Geometry: final body of the model. Coordinates: model frame, mm. A direction names the side the tool comes from. Round coordinates to 2 decimals unless told otherwise and drop trailing zeros. Loops run counter-clockwise (first coordinate to the right, second up) from the corner with the lowest first, then second, coordinate; pieces in that order, holes last. Notation, with made-up numbers: (-38, -13.5) - (-19, -13.5) arc R28 cw to (-19, 20.5) - close; hole circle Ø2 at (-27, -39.75). An arc over 180 degrees is marked (long way). Answer as a JSON object with one key per item and string values. Group by question number.
Item 1: Section B-B (z = 32). Return the cut outline in (x, y).
Item 2: Draft query along Y for faces 1 (the face through (-22.804, 25.315, 2.994)), 2 (the face through (-22.804, 21.115, 2.994)), 3 (the face through (-39.05, 1.97, -8.67)), 4 (the face through (0, 4, 3)). Return one class per face: released by +Y, released by -Y, zero draft, split by the parting line, or undercut.
Item 3: Section A-A (y = 7.25). Return the cut outline in (x, z).
Item 4: Line query: line 1 (X direction, y = 8.5, z = 0); line 2 (X direction, y = 1, z = 0); line 3 (Y direction, x = -6, z = -22.5). Output: solid intervals per line, ascending.
Item 5: First-contact query: pin 1 (3 mm diameter, centred on y = 14, z = 16.5, fed in from -X); pin 2 (3 mm diameter, centred on y = 19.5, z = -3.5, fed in from +X); pin 3 (16 mm diameter, centred on x = 0, z = 0, fed in from +Y). Flat tips, straight axial feed; report the tip coordinate or a pass-through.
Item 6: Reachability of faces 5 (the face through (7.21, 27.19, 22.89)), 6 (the face through (-12.93, 30, 11.3)) from +Z, -Z, +X, -X, +Y, -Y: full face, straight path, thin tool, end or side. Return the list, or none.
```python
from build123d import *

# Parameters (mm, degrees)
SKETCH1_R           = 40
SKETCH1_R_2         = 2.1
BOSS_EXTRUDE1_DEPTH = 4
SKETCH2_R           = 25
SKETCH2_R_2         = 6.1
BOSS_EXTRUDE5_DEPTH = 9
SKETCH6_R           = 22
SKETCH6_R_2         = 17
BOSS_EXTRUDE6_DEPTH = 5
SKETCH7_R           = 24
SKETCH7_R_2         = 17
BOSS_EXTRUDE7_DEPTH = 12
SKETCH9_W           = 1
SKETCH9_H           = 2.2
CHAMFER1_SIZE       = 2
FILLET1_R           = 2


with BuildPart() as part:
    # Sketch1 → Boss-Extrude1 (new body)
    with BuildSketch(Plane(origin=(0, 0, 0), x_dir=(1, 0, 0), z_dir=(0, 1, 0))):
        with Locations(Location((0, 0, 0), (0, 0, 270))):
            Circle(SKETCH1_R)
        with Locations(Location((0, 0, 0), (0, 0, 270))):
            Circle(SKETCH1_R_2, mode=Mode.SUBTRACT)
    extrude(amount=BOSS_EXTRUDE1_DEPTH)

    # Sketch2 → Boss-Extrude5 (add)
    with BuildSketch(Plane(origin=(0, 4, 0), x_dir=(1, 0, 0), z_dir=(0, 1, 0))):
        with Locations(Location((0, 0, 0), (0, 0, 270))):
            Circle(SKETCH2_R)
        with Locations(Location((0, 0, 0), (0, 0, 270))):
            Circle(SKETCH2_R_2, mode=Mode.SUBTRACT)
    extrude(amount=BOSS_EXTRUDE5_DEPTH)

    # Sketch6 → Boss-Extrude6 (add)
    with BuildSketch(Plane(origin=(0, 13, 0), x_dir=(1, 0, 0), z_dir=(0, 1, 0))):
        with Locations(Location((0, 0, 0), (0, 0, 270))):
            Circle(SKETCH6_R)
        with Locations(Location((0, 0, 0), (0, 0, 270))):
            Circle(SKETCH6_R_2, mode=Mode.SUBTRACT)
    extrude(amount=BOSS_EXTRUDE6_DEPTH)

    # Sketch7 → Boss-Extrude7 (add)
    with BuildSketch(Plane(origin=(0, 18, 0), x_dir=(1, 0, 0), z_dir=(0, 1, 0))):
        with Locations(Location((0, 0, 0), (0, 0, 270))):
            Circle(SKETCH7_R)
        with Locations(Location((0, 0, 0), (0, 0, 270))):
            Circle(SKETCH7_R_2, mode=Mode.SUBTRACT)
    extrude(amount=BOSS_EXTRUDE7_DEPTH)

    # Sketch9 → Cut-Revolve1 (revolve, cut)
    with BuildSketch(Plane(origin=(0, 0, 0), x_dir=(0, 0, -1), z_dir=(1, 0, 0)), mode=Mode.PRIVATE) as cut_revolve1_sk:
        with Locations((-23.5, 25.3)):
            Rectangle(SKETCH9_W, SKETCH9_H)
        with Locations((-23.5, 21.1)):
            Rectangle(SKETCH9_W, SKETCH9_H)
    revolve(cut_revolve1_sk.sketch.rotate(Axis((0, 0, 0), (0, 1, 0)), 180), axis=Axis((0, 0, 0), (0, 1, 0)), mode=Mode.SUBTRACT)

    # Chamfer1
    chamfer1_edges = [part.edges().sort_by_distance(p)[0] for p in [
        (0, 30, -24),
    ]]
    chamfer(chamfer1_edges, length=CHAMFER1_SIZE)

    # Fillet1
    fillet1_edges = [part.edges().sort_by_distance(p)[0] for p in [
        (0, 18, -22),
        (0, 13, -22),
    ]]
    fillet(fillet1_edges, radius=FILLET1_R - 0.0001)  # a hair under: the kernel refuses the full size


solid = part.part
```
Values:
{
 "1": {"outline": "(-24, 0) - (24, 0) - (24, 4) - (-24, 4) - close"},
 "2": {"face 1": "undercut", "face 2": "undercut", "face 3": "zero draft", "face 4": "released by +Y"},
 "3": {"outline": "circle Ø50 at (0, 0); hole circle Ø12.2 at (0, 0)"},
 "4": {"line 1": "x = -25 to -6.1, 6.1 to 25", "line 2": "x = -40 to -2.1, 2.1 to 40", "line 3": "y = 0 to 13.13, 17.87 to 20, 22.2 to 24.2, 26.4 to 28.71"},
 "5": {"pin 1": "stops at x = -19.71", "pin 2": "stops at x = 23.92", "pin 3": "stops at y = 13"},
 "6": {"face 5": "+Y", "face 6": "+Z, -Z, +X, -X, +Y"}
}
